Here's how the part is built. I have some questions about the finished solid (model axes, mm). Face numbers are marked on the shaded views. A direction names the side the tool comes from. Give positions to 0.01 mm unless a question says otherwise; leave off trailing zeros. Loops run counter-clockwise (first coordinate to the right, second up) from the corner with the lowest first, then second, coordinate; pieces in that order, holes last. Notation, with made-up numbers: M 68.5,37 L 114.5,37 A29 cw 114.5,59 Z; hole C 85.25,-33.75 d1. An arc over 180 degrees is marked long. Answer as CSV lines item,"result". Start each with the question number.
Item 1: If we mould it in two halves opening along Y, with no side actions, what happens to the marked faces 4, 5 and 6? For each: released by +Y, released by -Y, zero draft, split by the parting line, or undercut.
Item 2: If I drill on line 1 along X through (y, z) = (-6.5, -8) (3 decimals); line 2 along X through (y, z) = (-9, 1); line 3 along X through (y, z) = (-2.5, -4.75) (3 decimals), over which ranges is the centre line in solid material (lowest first)? Write a range as from..to.
Item 3: I want a section at C-C on z = 7.25. Give the number of separate pieces and of enclosed holes in the cut face, plus the area to 3 significant figures.
Item 4: For the marked faces 1, 2 and 3, which set-ups out of +Z, -Z, +X, -X, +Y, -Y let a thin tool reach every point of the face, with its end or its side?
Item 5: I want a section at A-A on x = 25.4. List the corners of the cut face in (y, z) for me.
Item 6: Will these pins go through, and if not, where does the flat tip stop? P1, Ø4, axis at x = -30.48, y = -5.588, coming from the +Z side; P2, Ø6, axis at x = 1.5, y = -6, coming from the -Z side; P3, Ø5, axis at x = 25.4, z = 6.36, coming from the +Y side; P4, Ø1, axis at y = -8, z = 5, coming from the +X side.
Item 7: I want a section at B-B on z = -7.5. List the corners of the cut face in (x, y) for me (3 decimals).
from build123d import *

# Parameters (mm, degrees)
F1_DEPTH       = 11.176
F2_R           = 3.175
F5_D           = 3.4544
F5_START       = 10.33145
F5_CBORE_D     = 6.35
F5_CBORE_DEPTH = 11.7602
F6_T1_DEPTH    = 43.8363739472
F8_D           = 7.9375
F10_D          = 3.175


# Not quite as in the source:
# - a fillet or chamfer that OpenCascade refuses, or shapes differently, is made with other operations: its cross-section is extruded or revolved along the edge and cut away or added


with BuildPart() as f1:
    # F0 (on Front) → F1 (new body)
    with BuildSketch(Plane.XZ):
        Polygon((38.1, 10.31875), (-38.1, 10.31875), (-38.1, -10.31875), (-22.225, -10.31875), (-22.225, -1.42875), (22.225, -1.42875), (22.225, -10.31875), (38.1, -10.31875), align=None)
    extrude(amount=F1_DEPTH)

    # F2
    f2_edges = [f1.edges().sort_by_distance(p)[0] for p in [
        (-22.225, -5.588, -1.42875),
        (22.225, -5.588, -1.42875),
    ]]
    fillet(f2_edges, radius=F2_R)

    # F5 (through all)
    # its depths count from where the whole tool has entered the part; down to there all is cleared
    with Locations(Plane.XY.offset(20.6502).offset(-F5_START)):
        with Locations((-30.48, -5.588), (30.48, -5.588)):
            CounterBoreHole(F5_D / 2, F5_CBORE_D / 2, F5_CBORE_DEPTH)

    # F6: chamfer of 6.35 on 2 edges, made by hand

    # F6_s2 → F6_t1 (cut)
    with BuildSketch(Plane.XZ.offset(-16.3301869736)):
        Polygon((-38.1, 3.96875), (-31.75, 10.31875), (-38.1, 10.31875), align=None)
        Polygon((31.75, 10.31875), (38.1, 3.96875), (38.1, 10.31875), align=None)
    extrude(amount=F6_T1_DEPTH, mode=Mode.SUBTRACT)

    # F8 (through all)
    with Locations(Plane.XY.offset(20.6502)):
        with Locations((-12.7, -5.588), (12.7, -5.588)):
            Hole(F8_D / 2)

    # F10 (through all)
    with Locations(Plane.XZ.offset(11.176)):
        with Locations((-25.4, 6.35635), (25.4, 6.35635)):
            Hole(F10_D / 2)


solid = f1.part
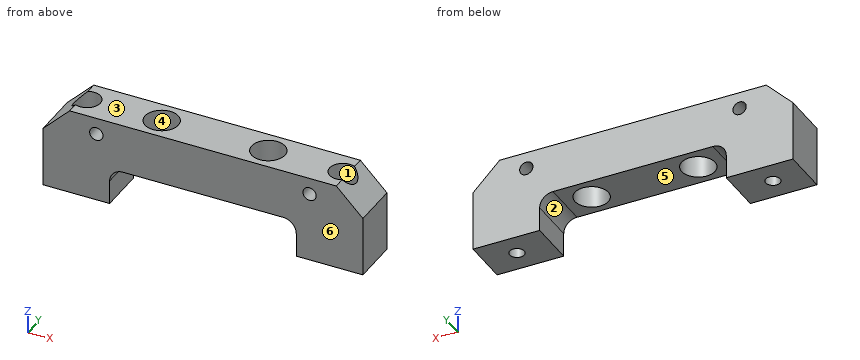
Result:
1,face 4,"undercut"
1,face 5,"zero draft"
1,face 6,"released by -Y"
2,line 1,"-38.1..-31.947, -29.013..-22.225, 22.225..29.013, 31.947..38.1"
2,line 2,"-38.1..-14.73, -10.67..10.67, 14.73..38.1"
2,line 3,"-38.1..-22.225, 22.225..38.1"
3,separate pieces,"3"
3,enclosed holes,"4"
3,area,"557 mm^2"
4,face 1,"+Z"
4,face 2,"-Z, +Y, -Y"
4,face 3,"+Z, +X, -X, +Y, -Y"
5,outline,"M -11.18,-10.32 L 0,-10.32 L 0,4.77 L -11.18,4.77 Z; M -11.18,7.94 L 0,7.94 L 0,10.32 L -11.18,10.32 Z"
6,P1,"z = -1.44"
6,P2,"z = -1.43"
6,P3,"y = 0"
6,P4,"x = 37.57"
7,outline,"M -38.1,-11.176 L -22.225,-11.176 L -22.225,0 L -38.1,0 Z; M 22.225,-11.176 L 38.1,-11.176 L 38.1,0 L 22.225,0 Z; hole C -30.48,-5.588 d3.454; hole C 30.48,-5.588 d3.454"
